Input: dimensioned drawing with shaded views. Units: mm. Origin: part minimum x, y, z. Coordinates: 2 decimals unless noted, no trailing zeros. Order: outer loops, then holes, each group sorted by start corner. A loop starts at its lowest first (then second) coordinate and runs counter-clockwise, first axis right, second up. Notation, with made-up numbers: M 15.25,-26 L 63.25,-26 A12 cw 63.25,-15 Z; hole C 43.5,88 d9. An arc over 180 degrees is marked long. Use CSV: the item, a comma, the result in double quotes. Start each with the question number.
1. Section query B-B on x = 203.5. Return the cut outline in (y, z).
2. First-contact query: P1, Ø5, axis at x = 54.95, z = 55, coming from the +Y side; P2, Ø1, axis at y = 4, z = 271, coming from the -X side; P3, Ø2, axis at x = 39.5, y = 3, coming from the -Z side; P4, Ø2.5, axis at y = 3.5, z = 290.5, coming from the +X side (3 decimals). Flat tips, straight axial feed; report the tip coordinate or a pass-through.
3. Section query A-A on y = 1.8. State how many separate pieces and enclosed holes the cut face has, and give its area (3 significant figures).
4. Material intervals for line 1 (X direction, y = 1.65, z = 265) (1 decimal); line 2 (Z direction, x = 176, y = 2.1); line 3 (X direction, y = 1.1, z = 19) (1 decimal), sorted ascending.
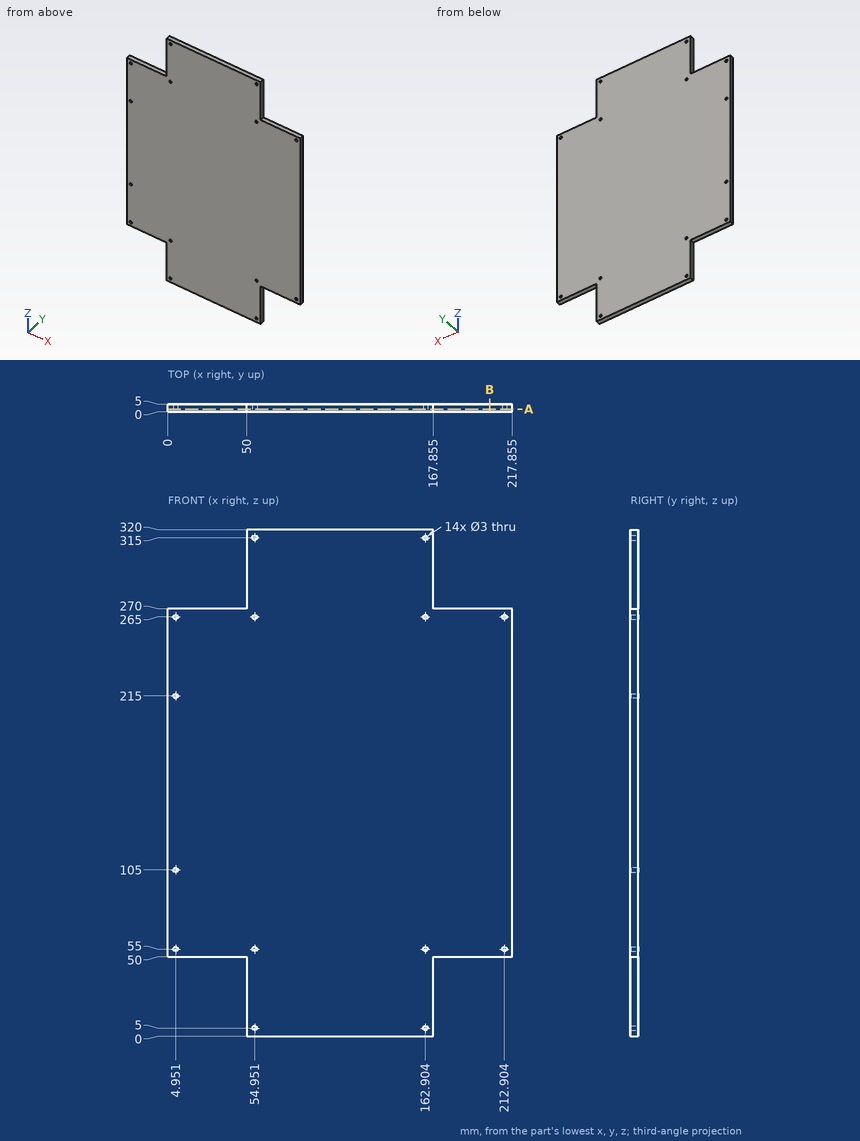
Results list:
1,outline,"M 0,50 L 5,50 L 5,270 L 0,270 Z"
2,P1,"stops at y = 5"
2,P2,"stops at x = 50"
2,P3,"stops at z = 50"
2,P4,"stops at x = 167.855"
3,separate pieces,"1"
3,enclosed holes,"14"
3,area,"59,600 mm²"
4,line 1,"x = 0 to 3.5, 6.5 to 53.5, 56.5 to 161.4, 164.4 to 211.4, 214.4 to 217.9"
4,line 2,"z = 50 to 270"
4,line 3,"x = 50 to 167.9"
